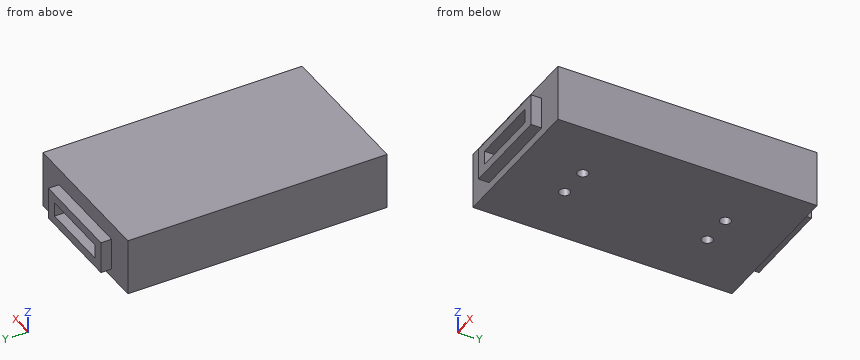
```python
from build123d import *

# Parameters (mm, degrees)
SKETCH_W          = 42
SKETCH_H          = 16
PAD_DEPTH         = 36.35
SKETCH001_W       = 26
SKETCH001_H       = 9
PAD001_DEPTH      = 39.35
SKETCH002_W       = 20
SKETCH002_H       = 4
POCKET_DEPTH      = 39.351
POCKET_DEPTH_BACK = -39.351
SKETCH003_R       = 1.5
POCKET001_DEPTH   = 5


with BuildPart() as part:
    # Sketch → Pad (new body, symmetric)
    with BuildSketch(Plane.XZ):
        with Locations((0, 8)):
            Rectangle(SKETCH_W, SKETCH_H)
    extrude(amount=PAD_DEPTH, both=True)

    # Sketch001 → Pad001 (join, symmetric)
    with BuildSketch(Plane.XZ):
        with Locations((0, 6.9)):
            Rectangle(SKETCH001_W, SKETCH001_H)
    extrude(amount=PAD001_DEPTH, both=True)

    # Sketch002 → Pocket (cut, two sides)
    with BuildSketch(Plane.XZ) as pocket_sk:
        with Locations((0, 6.9)):
            Rectangle(SKETCH002_W, SKETCH002_H)
    extrude(amount=-POCKET_DEPTH, mode=Mode.SUBTRACT)
    extrude(pocket_sk.sketch, amount=-POCKET_DEPTH_BACK, mode=Mode.SUBTRACT)

    # Sketch003 → Pocket001 (cut)
    with BuildSketch(Plane.XY):
        with Locations((-4.5, 20)):
            Circle(SKETCH003_R)
        with Locations((4.5, 20)):
            Circle(SKETCH003_R)
        with Locations((-4.5, -20)):
            Circle(SKETCH003_R)
        with Locations((4.5, -20)):
            Circle(SKETCH003_R)
    extrude(amount=POCKET001_DEPTH, mode=Mode.SUBTRACT)


solid = part.part
```
Check sheet for the modelled part. Datum: model origin and axes. Units: mm. Coordinates: 2 decimals unless noted, no trailing zeros. Order: outer loops, then holes, each group sorted by start corner. A loop starts at its lowest first (then second) coordinate and runs counter-clockwise, first axis right, second up. Notation, with made-up numbers: M -4,30.25 L 41,30.25 A27 ccw 41,56.25 Z; hole C 36.25,82 d10. An arc over 180 degrees is marked long. Write each question's results on one line, items separated by ' | '. Start each with the question number.
1. Cross-section at D-D on x = 18.5. Record the cut outline in (y, z).
2. Cross-section at A-A on x = 4.5. Record the cut outline in (y, z), and give its area (3 significant figures).
3. Cross-section at B-B on y = 20. Record the cut outline in (x, z).
4. Go/stop test with flat-tipped pins: P1, Ø3.5, axis at y = -38, z = 5.5, coming from the -X side; P2, Ø1.5, axis at x = -4.5, z = 7, coming from the -Y side; P3, Ø1.8, axis at x = 4.5, y = 20, coming from the -Z side; P4, Ø1.5, axis at x = 1.5, y = -38, coming from the +Z side. Record where each tip stops, or that it passes through.
5. Material ranges on probe 1 along Y at (x, z) = (-4.5, 1.75); probe 2 along Y at (x, z) = (4.5, 3.6); probe 3 along Z at (x, y) = (-3, 32), recorded low to high.
6. Cross-section at C-C on y = -26.5. Record the cut outline in (x, z).
Checks:
1) outline: M -36.35,0 L 36.35,0 L 36.35,16 L -36.35,16 Z
2) outline: M -39.35,2.4 L -36.35,2.4 L -36.35,0 L -21.5,0 L -21.5,4.9 L -39.35,4.9 Z; M -39.35,8.9 L 39.35,8.9 L 39.35,11.4 L 36.35,11.4 L 36.35,16 L -36.35,16 L -36.35,11.4 L -39.35,11.4 Z; M -18.5,0 L 18.5,0 L 18.5,4.9 L -18.5,4.9 Z; M 21.5,0 L 36.35,0 L 36.35,2.4 L 39.35,2.4 L 39.35,4.9 L 21.5,4.9 Z | area: 873 mm²
3) outline: M -21,0 L -6,0 L -6,4.9 L -10,4.9 L -10,8.9 L 10,8.9 L 10,4.9 L 6,4.9 L 6,0 L 21,0 L 21,16 L -21,16 Z; M -3,0 L 3,0 L 3,4.9 L -3,4.9 Z
4) P1: stops at x = -21 | P2: passes through | P3: stops at z = 8.9 | P4: stops at z = 11.4
5) probe 1: y = -36.35 to -21.5, -18.5 to 18.5, 21.5 to 36.35 | probe 2: y = -39.35 to -21.5, -18.5 to 18.5, 21.5 to 39.35 | probe 3: z = 0 to 4.9, 8.9 to 16
6) outline: M -21,0 L 21,0 L 21,16 L -21,16 Z; hole M -10,4.9 L 10,4.9 L 10,8.9 L -10,8.9 Z
